from build123d import *

# Parameters (mm, degrees)
SKETCH1_W           = 76.454565701
SKETCH1_H           = 16.829621381
BOSS_EXTRUDE1_DEPTH = 1
SKETCH3_W           = 76
SKETCH3_H           = 14.736718314
BOSS_EXTRUDE2_DEPTH = 10
SCALE1_SCALE        = 0.2


with BuildPart() as part:
    # Sketch1 → Boss-Extrude1 (new body)
    with BuildSketch(Plane(origin=(0, 0, 0), x_dir=(1, 0, 0), z_dir=(0, 1, 0))):
        with Locations((-6.298094695, 43.757015591)):
            Rectangle(SKETCH1_W, SKETCH1_H)
    extrude(amount=BOSS_EXTRUDE1_DEPTH)

    # Sketch3 → Boss-Extrude2 (add)
    with BuildSketch(Plane(origin=(0, 0, 0), x_dir=(1, 0, 0), z_dir=(0, 1, 0))):
        with Locations((-6.386632835, 43.82550718)):
            Rectangle(SKETCH3_W, SKETCH3_H)
    extrude(amount=BOSS_EXTRUDE2_DEPTH)


with BuildPart() as part_1:
    # Scale1: scaled about (-6.376610315, 4.933999832, -43.81775393)
    add(part.part.scale(SCALE1_SCALE).moved(Location((-5.101288252, 3.947199866, -35.054203144))))


solid = part_1.part
Check sheet for the modelled part. Datum: model origin and axes. Units: mm. A direction names the side the tool comes from. Coordinates: 2 decimals unless noted, no trailing zeros. Write each loop counter-clockwise with the first axis right and the second up, starting at its lowest first coordinate (ties: lowest second). Pieces come first, ordered by that corner, then holes. Notation, with made-up numbers: M 44,7.25 L 52,7.25 A19 ccw 52,41.25 Z; hole C -38.75,61.25 d1. An arc over 180 degrees is marked long. Answer as CSV lines item,"result".
Q1. Set-up check for faces 1 (the face through (-6, 5.947, -44)), 2 (the face through (-6, 5, -42.346)): record each of +Z, -Z, +X, -X, +Y, -Y from which the full face is reachable in a straight line by a thin tool's end or side.
Check result:
face 1,"+Z, -Z, +X, -X, +Y"
face 2,"+Z, +X, -X, +Y"
Q2. Material ranges on probe 1 along X at (y, z) = (4.75, -43.45); probe 2 along Z at (x, y) = (-5, 4.9); probe 3 along Y at (x, z) = (-8.25, -42.3), recorded low to high. Write a range as from..to.
Check result:
probe 1,"-13.98..1.22"
probe 2,"-45.29..-42.35"
probe 3,"3.95..4.15"
Q3. Mould release check, pull along X, two halves, no side actions. Record for faces 3 (the face through (-6, 5, -45.293)), 4 (the face through (-13.979, 5, -44)), 5 (the face through (1.221, 5, -44)): released by +X, released by -X, zero draft, split by the parting line, or undercut.
Check result:
face 3,"zero draft"
face 4,"released by -X"
face 5,"released by +X"
Q4. Cross-section at B-B (y = 5.3). Record the boundary of the cut face in (x, z).
Check result:
outline,"M -13.98,-45.29 L 1.22,-45.29 L 1.22,-42.35 L -13.98,-42.35 Z"
Q5. Cross-section at A-A (x = -5.5). Record the boundary of the cut face in (y, z), then the cut area to 3 significant figures.
Check result:
outline,"M 3.95,-45.49 L 4.15,-45.49 L 4.15,-45.29 L 5.95,-45.29 L 5.95,-42.35 L 4.15,-42.35 L 4.15,-42.12 L 3.95,-42.12 Z"
area,"5.98 mm^2"
Q6. Go/stop test with flat-tipped pins: pin 1 (0.5 mm diameter, centred on y = 5, z = -43.5, fed in from +X); pin 2 (1 mm diameter, centred on y = 5.5, z = -42.5, fed in from -X). Record where each tip stops, or that it passes through.
Check result:
pin 1,"x = 1.22"
pin 2,"x = -13.98"
